Could you check a few things on this model? Use its own coordinates, in mm. A direction names the side the tool comes from. Round coordinates to 2 decimals unless told otherwise and drop trailing zeros. Write each loop counter-clockwise with the first axis right and the second up, starting at its lowest first coordinate (ties: lowest second). Pieces come first, ordered by that corner, then holes. Notation, with made-up numbers: (30.25, -1.5) -> (76.25, -1.5) arc R14 cw to (76.25, 6.5) -> close; hole circle Ø1 at (89.5, 43). An arc over 180 degrees is marked (long way). Answer in a Markdown table with one row per item.
from build123d import *

# Parameters (mm, degrees)
BOSS_EXTRUDE1_DEPTH = 444.5
BOSS_EXTRUDE2_DEPTH = 25.4


with BuildPart() as part:
    # Sketch1 → Boss-Extrude1 (new, symmetric)
    with BuildSketch(Plane(origin=(0, 0, 0), x_dir=(0, 0, -1), z_dir=(1, 0, 0))):
        with BuildLine():
            Line((12.7, 31.75), (12.7, -31.75))
            ThreePointArc((12.7, -31.75), (0, -44.45), (-12.7, -31.75))
            Line((-12.7, -31.75), (-12.7, 31.75))
            ThreePointArc((-12.7, 31.75), (0, 44.45), (12.7, 31.75))
        make_face()
    extrude(amount=BOSS_EXTRUDE1_DEPTH, both=True)

    # Sketch2 → Boss-Extrude2 (add)
    with BuildSketch(Plane(origin=(444.5, 0, 0), x_dir=(0, 0, -1), z_dir=(1, 0, 0))):
        with BuildLine():
            Line((-6.35, -25.4), (-6.35, 25.4))
            ThreePointArc((-6.35, 25.4), (0, 31.75), (6.35, 25.4))
            Line((6.35, 25.4), (6.35, -25.4))
            ThreePointArc((6.35, -25.4), (0, -31.75), (-6.35, -25.4))
        make_face()
    boss_extrude2 = extrude(amount=BOSS_EXTRUDE2_DEPTH)

    # Mirror1: Boss-Extrude2 across plane
    add(boss_extrude2.mirror(Plane(origin=(0, 0, 0), x_dir=(0, 0, 1), z_dir=(1, 0, 0))))


solid = part.part
1) Imagine slicing it at C-C, the plane x = -2. Please give me the cut outline in (y, z).
Findings:
| item | result |
|---|---|
| outline | (-31.75, -12.7) -> (31.75, -12.7) arc R12.7 ccw to (31.75, 12.7) -> (-31.75, 12.7) arc R12.7 ccw to start |
2) For pin 1 (7.5 mm diameter, centred on x = -455, y = 11, fed in from +Z); pin 2 (8 mm diameter, centred on x = 223.5, z = -6, fed in from -Y); pin 3 (12 mm diameter, centred on x = 335.5, z = -9, fed in from -Y), each with a flat end and sliding along its axis, tell me the tip position at first contact or that it passes through.
Findings:
| item | result |
|---|---|
| pin 1 | stops at z = 6.35 |
| pin 2 | stops at y = -44.29 |
| pin 3 | stops at y = -44.09 |
3) Please list where these lines run through material, in increasing order: line 1 (X direction, y = -5, z = -8.75); line 2 (Y direction, x = 44.5, z = 1.25); line 3 (Y direction, x = 194, z = -2).
Findings:
| item | result |
|---|---|
| line 1 | x = -444.5 to 444.5 |
| line 2 | y = -44.39 to 44.39 |
| line 3 | y = -44.29 to 44.29 |
4) For faces 1 (the face through (-457, 0, -6.35)), 2 (the face through (457, 0, 6.35)), 3 (the face through (444.5, 1, 8)), 4 (the face through (457, 0, -6.35)), which set-ups out of +Z, -Z, +X, -X, +Y, -Y let a thin tool reach every point of the face, with its end or its side?
Findings:
| item | result |
|---|---|
| face 1 | -Z, -X, +Y, -Y |
| face 2 | +Z, +X, +Y, -Y |
| face 3 | +X |
| face 4 | -Z, +X, +Y, -Y |
5) Imagine slicing it at B-B, the plane z = 0. Please give me the cut outline in (x, y).
Findings:
| item | result |
|---|---|
| outline | (-469.9, -31.75) -> (-444.5, -31.75) -> (-444.5, -44.45) -> (444.5, -44.45) -> (444.5, -31.75) -> (469.9, -31.75) -> (469.9, 31.75) -> (444.5, 31.75) -> (444.5, 44.45) -> (-444.5, 44.45) -> (-444.5, 31.75) -> (-469.9, 31.75) -> close |
6) Imagine slicing it at A-A, the plane y = 6. Please give me the cut outline in (x, z).
Findings:
| item | result |
|---|---|
| outline | (-469.9, -6.35) -> (-444.5, -6.35) -> (-444.5, -12.7) -> (444.5, -12.7) -> (444.5, -6.35) -> (469.9, -6.35) -> (469.9, 6.35) -> (444.5, 6.35) -> (444.5, 12.7) -> (-444.5, 12.7) -> (-444.5, 6.35) -> (-469.9, 6.35) -> close |
7) Thinking about a two-plate mould opening in Y: for faces 5 (the face through (6.223, 44.447, 0.279)), 6 (the face through (-457, 0, 6.35)), 7 (the face through (6.223, -44.447, -0.279)), which applies, +Y half, -Y half, draft (parallel to the pull), parting line (faces both ways), or undercut?
Findings:
| item | result |
|---|---|
| face 5 | +Y half |
| face 6 | draft |
| face 7 | -Y half |
